```python
from build123d import *

# Parameters (mm, degrees)
CHAMFER_1_SIZE               = 2.5
CHAMFER_1_SIZE2              = 4.330127019
CHAMFER_2_SIZE               = 1
CHAMFER_2_SIZE2              = 1.732050808
HOLE_WIZARD_M6_1_D           = 5
HOLE_WIZARD_M6_1_DEPTH       = 8
HOLE_WIZARD_M6_1_CSINK_D     = 8
HOLE_WIZARD_M6_1_CSINK_ANGLE = 90
HOLE_WIZARD_M6_1_TIP         = 1.502151548
SKETCH_4_R                   = 1.5
CUT_EXTRUDE_1_DEPTH          = 20


with BuildPart() as part:
    # 草图1 (on Front Plane) → 旋转1 (revolve)
    with BuildSketch(Plane.XY, mode=Mode.PRIVATE) as revolve_1_sk:
        Polygon((0, 0), (0, 12.5), (-7, 12.5), (-7, 17), (-32, 17), (-32, 14), (-10, 14), (-10, 0), align=None)
    revolve(revolve_1_sk.sketch.rotate(Axis((-10, 0, 0), (1, 0, 0)), 90), axis=Axis((-10, 0, 0), (1, 0, 0)))

    # 倒角1
    chamfer_1_edges = [part.edges().sort_by_distance(p)[0] for p in [
        (0, 0, -12.5),
    ]]
    chamfer_1_side = [part.faces().sort_by_distance(p)[0] for p in [
        (0, 0, 0),
    ]]
    chamfer(chamfer_1_edges, length=CHAMFER_1_SIZE, length2=CHAMFER_1_SIZE2, reference=chamfer_1_side[0])

    # 倒角2
    chamfer_2_edges = [part.edges().sort_by_distance(p)[0] for p in [
        (-7, 0, -17),
    ]]
    chamfer_2_side = [part.faces().sort_by_distance(p)[0] for p in [
        (-7, 0, -12.980832611),
    ]]
    chamfer(chamfer_2_edges, length=CHAMFER_2_SIZE, length2=CHAMFER_2_SIZE2, reference=chamfer_2_side[0])

    # M6 螺纹孔1
    with Locations(Plane(origin=(-10, 0, 0), x_dir=(0, 0, -1), z_dir=(-1, 0, 0))):
        with Locations((0, 0)):
            CounterSinkHole(HOLE_WIZARD_M6_1_D / 2, HOLE_WIZARD_M6_1_CSINK_D / 2, depth=HOLE_WIZARD_M6_1_DEPTH, counter_sink_angle=HOLE_WIZARD_M6_1_CSINK_ANGLE)
            with Locations((0, 0, -(HOLE_WIZARD_M6_1_DEPTH + HOLE_WIZARD_M6_1_TIP / 2))):  # 118° drill point
                Cone(0, HOLE_WIZARD_M6_1_D / 2, HOLE_WIZARD_M6_1_TIP, mode=Mode.SUBTRACT)

    # 草图4 → 切除-拉伸1 (cut, symmetric)
    with BuildSketch(Plane(origin=(0, 0, 0), x_dir=(1, 0, 0), z_dir=(0, 1, 0))):
        with Locations(Location((-12, 0, 0), (0, 0, 270))):
            Circle(SKETCH_4_R)
    extrude(amount=CUT_EXTRUDE_1_DEPTH, both=True, mode=Mode.SUBTRACT)


solid = part.part
```
Build history of the part. All positions in model axes, mm. A direction names the side the tool comes from. Round coordinates to 2 decimals unless told otherwise and drop trailing zeros. Write each loop counter-clockwise with the first axis right and the second up, starting at its lowest first coordinate (ties: lowest second). Pieces come first, ordered by that corner, then holes. Notation, with made-up numbers: (37, 83.5) -> (64, 83.5) arc R38 ccw to (64, 122.5) -> close; hole circle Ø4 at (25.5, 52.5). An arc over 180 degrees is marked (long way). Put each result on its own line as item: value.
Item 1: Flat gauge pins, fed straight in: P1, Ø8.5, axis at y = -0.5, z = -7, coming from the -X side; P2, Ø4, axis at x = -5.5, y = 4, coming from the +Z side; P3, Ø2, axis at x = -3.5, y = 7, coming from the -Z side. Where does each tip first touch, or does it go through?
Here are the results:
P1: stops at x = -10
P2: stops at z = 15.88
P3: stops at z = -10.72
Item 2: Wall check: probe 1 along X at (y, z) = (-14.8, 0); probe 2 along Y at (x, z) = (-6, 0); probe 3 along Y at (x, z) = (-15.75, 0). Give the ranges that are in metal, low to high. Write a range as from..to.
Here are the results:
probe 1: x = -32..-13.5, -10.5..-7
probe 2: y = -12.5..-2.5, 2.5..12.5
probe 3: y = -17..-14, 14..17
Item 3: Slice it at B-B, the plane x = -27.5. Give the cut face in (y, z), plus the area to 3 significant figures.
Here are the results:
outline: circle Ø34 at (0, 0); hole circle Ø28 at (0, 0)
area: 292 mm^2
Item 4: Tool access for faces 1 (the face through (-20.8, 12.4, 6.5)), 2 (the face through (-20.529, -16.855, -2.213)): list every direction of +Z, -Z, +X, -X, +Y, -Y with a clear straight run to the whole face (end or side of a thin tool).
Here are the results:
face 1: -X
face 2: +X, -X
Item 5: Two-plate mould, pull along X, no slides. Class faces 3 (the face through (-11.55, 15.48, 1.43)), 4 (the face through (-5.684, -3.755, 11.923)), 5 (the face through (-11.55, -15.44, 1.43)), 6 (the face through (-7, 8, 10)): pulls with the +X half, pulls with the -X half, needs draft (parallel to the pull), parting line crosses it, or undercut.
Here are the results:
face 3: undercut
face 4: needs draft
face 5: undercut
face 6: pulls with the +X half
